Check sheet for the modelled part. Datum: model origin and axes. Units: mm. A direction names the side the tool comes from. Give positions to 0.01 mm unless a question says otherwise; leave off trailing zeros. Order: outer loops, then holes, each group sorted by start corner. A loop starts at its lowest first (then second) coordinate and runs counter-clockwise, first axis right, second up. Notation, with made-up numbers: (57.5, 15.25) -> (81.5, 15.25) arc R24 cw to (81.5, 31.25) -> close; hole circle Ø8 at (43, 64.25). An arc over 180 degrees is marked (long way). One line per question, with ' | ' between items. Start each with the question number.
Autodesk Inventor part; units mm, degrees
ref_plane "YZ Plane" through (0, 0, 0) normal (1, 0, 0) x (0, 1, 0)
ref_plane "XZ Plane" through (0, 0, 0) normal (0, 1, 0) x (-1, 0, 0)
ref_plane "XY Plane" through (0, 0, 0) normal (0, 0, 1) x (1, 0, 0)
sketch "Skizze1" plane through (0, 0, 0) normal (0, 0, 1) x (1, 0, 0)
  circle A0 centre (0, 0) radius 3
  dimension "d0" = 6
extrude "Extrusion1" add sketch "Skizze1" along normal blind 21
hole "Bohrung1" at (0, 0, 21) direction (0, 0, -1) diameter 2.459 end through all
sketch "Skizze2" plane through (0, 0, 21) normal (0, 0, 1) x (1, 0, 0)
  circle A0 centre (0, 0) radius 3
  circle A1 centre (0, 0) radius 4
  dimension "d12" = 8
extrude "Extrusion2" add sketch "Skizze2" against normal blind 7
properties part number "13_0204_043"
1. Go/stop test with flat-tipped pins: pin 1 (1 mm diameter, centred on y = 3, z = 8.5, fed in from -X); pin 2 (1 mm diameter, centred on y = 2.5, z = 16, fed in from +X); pin 3 (2 mm diameter, centred on x = 0, y = 0, fed in from +Z); pin 4 (3 mm diameter, centred on x = -2, z = 9.5, fed in from +Y). Record where each tip stops, or that it passes through.
2. Cross-section at A-A on y = 0. Record the boundary of the cut face in (x, z).
3. Tool access check on faces 1 (the face through (1, 3, 14)), 2 (the face through (-1, -1, 21)). Record the directions out of +Z, -Z, +X, -X, +Y, -Y that give a thin tool (end or side, any length) a straight path to the whole face; none if there is none.
4. Cross-section at D-D on y = 2.25. Record the boundary of the cut face in (x, z).
5. Scan lines: probe 1 along Y at (x, z) = (0, 9); probe 2 along Z at (x, y) = (1.75, 2.5); probe 3 along X at (y, z) = (1, 16). Record each from-to range of solid material in increasing order.
6. Mould release check, pull along Y, two halves, no side actions. Record for faces 3 (the face through (-3, 0, 7)), 4 (the face through (1, -1, 0)), 5 (the face through (0.748, 0.976, 10.353)): +Y half, -Y half, draft (parallel to the pull), parting line (faces both ways), or undercut.
7. Cross-section at C-C on z = 19.5. Record the boundary of the cut face in (x, y), and give its area (3 significant figures).
Response values:
1) pin 1: stops at x = -1.66 | pin 2: stops at x = 3.46 | pin 3: passes through | pin 4: stops at y = 2.96
2) outline: (-4, 14) -> (-3, 14) -> (-3, 0) -> (-1.23, 0) -> (-1.23, 21) -> (-4, 21) -> close; (1.23, 0) -> (3, 0) -> (3, 14) -> (4, 14) -> (4, 21) -> (1.23, 21) -> close
3) face 1: -Z | face 2: +Z, +X, -X, +Y, -Y
4) outline: (-3.31, 14) -> (-1.98, 14) -> (-1.98, 0) -> (1.98, 0) -> (1.98, 14) -> (3.31, 14) -> (3.31, 21) -> (-3.31, 21) -> close
5) probe 1: y = -3 to -1.23, 1.23 to 3 | probe 2: z = 14 to 21 | probe 3: x = -3.87 to -0.72, 0.72 to 3.87
6) face 3: parting line | face 4: draft | face 5: undercut
7) outline: circle Ø8 at (0, 0); hole circle Ø2.46 at (0, 0) | area: 45.5 mm²
